For this review, take the finished solid that the model builds, in its own axes (mm). Give positions to 0.01 mm unless a question says otherwise; leave off trailing zeros. Write each loop counter-clockwise with the first axis right and the second up, starting at its lowest first coordinate (ties: lowest second). Pieces come first, ordered by that corner, then holes.
Q1. We need section B-B (y = 2.5). Write out the cut boundary in (x, z).
Q2. For line 1 (Y direction, x = 7, z = 1.5); line 2 (Y direction, x = 19, z = -5); line 3 (X direction, y = -27.5, z = 11), list the stretches that pass through material, from the lowest coordinate up.
Q3. Insertion check: P1, Ø10, axis at x = 20, z = 10.5, coming from the +Y side; P2, Ø2, axis at x = 15, z = 9.5, coming from the +Y side; P3, Ø12, axis at x = 8.5, z = 0.5, coming from the -Y side. Each pin has a flat end and moves straight along its axis. Give the tip position at first contact, or say it passes through.
Q4. We need section C-C (z = -3). Write out the cut boundary in (x, y), then the cut area to 3 significant figures.
```python
from build123d import *

# Parameters (mm, degrees)
F0_W     = 76.2
F0_H     = 55.5625
F1_DEPTH = 25.4
F2_R     = 55.56249
F4_DEPTH = 25.4
F6_DEPTH = 55.5635


# Not quite as in the source:
# - a fillet or chamfer is up to 0.001 mm smaller than in the source, because OpenCascade refuses the exact size


with BuildPart() as f1:
    # F0 (on Right) → F1 (new body)
    with BuildSketch(Plane.YZ):
        Rectangle(F0_W, F0_H)
    extrude(amount=F1_DEPTH)

    # F2 (radius 55.5625 in the source; OpenCascade refuses exactly that, so slightly less here)
    f2_edges = [f1.edges().sort_by_distance(p)[0] for p in [
        (12.7, 38.1, -27.78125),
    ]]
    fillet(f2_edges, radius=F2_R)

    # F3 (on face) → F4 (cut)
    with BuildSketch(Plane.YZ.offset(25.4)):
        with BuildLine():
            ThreePointArc((17.0539420908, 6.7351920908), (3.5835579092, 6.7351920908), (3.5835579092, -6.7351920908))
            Line((3.5835579092, -6.7351920908), (17.0539420908, 6.7351920908))
        make_face()
        with BuildLine():
            Line((17.0539420908, 6.7351920908), (3.5835579092, -6.7351920908))
            ThreePointArc((3.5835579092, -6.7351920908), (13.9638096933, -8.7999525472), (19.84375, 0))
            ThreePointArc((19.84375, 0), (19.1187025472, 3.6450596933), (17.0539420908, 6.7351920908))
        make_face()
    extrude(amount=-F4_DEPTH, mode=Mode.SUBTRACT)

    # F5 (on face) → F6 (cut, through all)
    with BuildSketch(Plane.XY.offset(27.78125)):
        Polygon((25.4, -12.7), (0, -38.1), (25.4, -38.1), align=None)
    extrude(amount=-F6_DEPTH, mode=Mode.SUBTRACT)


solid = f1.part
```
Computed:
1. outline: (0, -24.07) - (25.4, -24.07) - (25.4, -5.44) - (0, -5.44) - close; (0, 5.44) - (25.4, 5.44) - (25.4, 27.78) - (0, 27.78) - close
2. line 1: y = -31.1 to 0.91, 19.72 to 31.49
2. line 2: y = -19.1 to 2.21, 18.43 to 27.4
2. line 3: x = 0 to 10.6
3. P1: stops at y = 36.73
3. P2: stops at y = 35.34
3. P3: stops at y = -35.6
4. outline: (0, -38.1) - (25.4, -12.7) - (25.4, 1.28) - (0, 1.28) - close; (0, 19.36) - (25.4, 19.36) - (25.4, 28.79) - (0, 28.79) - close
4. area: 917 mm2
